The model under review builds one solid part; all positions refer to its coordinate system, in mm. Face numbers are marked on the shaded views. A direction names the side the tool comes from. Coordinates: 2 decimals unless noted, no trailing zeros. Write each loop counter-clockwise with the first axis right and the second up, starting at its lowest first coordinate (ties: lowest second). Pieces come first, ordered by that corner, then holes. Notation, with made-up numbers: M 51,68 L 83,68 A9 cw 83,84 Z; hole C 55,-38 d8. An arc over 180 degrees is marked long. Answer as a JSON object with one key per item and string values.
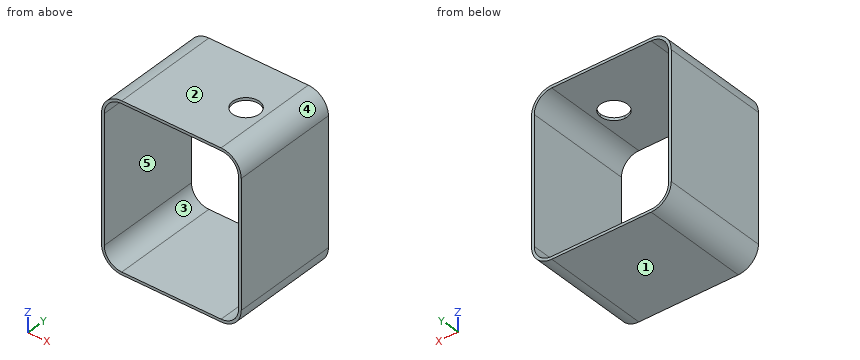
```python
from build123d import *

# Parameters (mm, degrees)
F1_DEPTH = 400
F3_DEPTH = 25


with BuildPart() as f1:
    # F0 (on Front) → F1 (new body)
    with BuildSketch(Plane.XZ):
        with BuildLine():
            Line((260, -235), (260, 235))
            ThreePointArc((260, 235), (238.033009, 288.033009), (185, 310))
            Line((185, 310), (-185, 310))
            ThreePointArc((-185, 310), (-238.033009, 288.033009), (-260, 235))
            Line((-260, 235), (-260, -235))
            ThreePointArc((-260, -235), (-238.033009, -288.033009), (-185, -310))
            Line((-185, -310), (185, -310))
            ThreePointArc((185, -310), (238.033009, -288.033009), (260, -235))
        make_face()
        with BuildLine():
            ThreePointArc((-250, 235), (-230.961941, 280.961941), (-185, 300))
            Line((-185, 300), (185, 300))
            ThreePointArc((185, 300), (230.961941, 280.961941), (250, 235))
            Line((250, 235), (250, -235))
            ThreePointArc((250, -235), (230.961941, -280.961941), (185, -300))
            Line((185, -300), (-185, -300))
            ThreePointArc((-185, -300), (-230.961941, -280.961941), (-250, -235))
            Line((-250, -235), (-250, 235))
        make_face(mode=Mode.SUBTRACT)
    extrude(amount=F1_DEPTH)

    # F2 (on face) → F3 (cut)
    with BuildSketch(Plane.XY.offset(310)):
        with BuildLine():
            ThreePointArc((165.524478, -200), (80.169139, -164.644661), (115.524478, -250))
            ThreePointArc((115.524478, -250), (150.879817, -235.355339), (165.524478, -200))
        make_face()
    extrude(amount=-F3_DEPTH, mode=Mode.SUBTRACT)


solid = f1.part
```
(1) For pin 1 Ø1 at (x, y) = (199.5, -165) entering from +Z; pin 2 Ø5 at (x, y) = (-206.5, -143) entering from +Z; pin 3 Ø1 at (x, y) = (-197.5, -116.5) entering from +Z, all flat-tipped, find the tip position at first contact; note any pin that passes through.
Results list:
{"pin 1": "z = 308.68", "pin 2": "z = 307.55", "pin 3": "z = 309.03"}
(2) Add section A-A on y = -138.5. Give the boundary of the cut face in (x, z).
Results list:
{"outline": "M -260,-235 A75 ccw -185,-310 L 185,-310 A75 ccw 260,-235 L 260,235 A75 ccw 185,310 L -185,310 A75 ccw -260,235 Z; hole M -250,-235 A65 ccw -185,-300 L 185,-300 A65 ccw 250,-235 L 250,235 A65 ccw 185,300 L -185,300 A65 ccw -250,235 Z"}
(3) For the marked faces 4 and 5, list the 3-axis set-ups (+Z, -Z, +X, -X, +Y, -Y) from which the entire face can be reached by the end or side of a thin tool; tool diameter is ignored.
Results list:
{"face 4": "+Z, +X, +Y, -Y", "face 5": "+Y, -Y"}
(4) Add section B-B on z = 24. Give the boundary of the cut face in (x, y).
Results list:
{"outline": "M -260,-400 L -250,-400 L -250,0 L -260,0 Z; M 250,-400 L 260,-400 L 260,0 L 250,0 Z"}
(5) Draft analysis for pull direction Z (two halves, no side actions). For the marked faces 1, 2 and 3, state which applies: released by +Z, released by -Z, zero draft, split by the parting line, or undercut.
Results list:
{"face 1": "released by -Z", "face 2": "released by +Z", "face 3": "undercut"}
(6) Add section D-D on x = 151. Give the boundary of the cut face in (y, z), and give its area (3 significant figures).
Results list:
{"outline": "M -400,-310 L 0,-310 L 0,-300 L -400,-300 Z; M -400,300 L -235.23,300 L -235.23,310 L -400,310 Z; M -164.77,300 L 0,300 L 0,310 L -164.77,310 Z", "area": "7,300 mm²"}
(7) Wall thickness on line 1 along X through (y, z) = (-258, -196.5); line 2 along Z through (x, y) = (-136.5, -280); line 3 along X through (y, z) = (-24.5, -273): over which ranges is each line inside the solid? List them lowest first. Write a range as from..to.
Results list:
{"line 1": "-260..-250, 250..260", "line 2": "-310..-300, 300..310", "line 3": "-249.66..-237.74, 237.74..249.66"}
(8) Add section C-C on x = 58. Give the boundary of the cut face in (y, z).
Results list:
{"outline": "M -400,-310 L 0,-310 L 0,-300 L -400,-300 Z; M -400,300 L 0,300 L 0,310 L -400,310 Z"}
